Check sheet for the drawn part. Datum: minimum x, y, z corner. Units: mm. A direction names the side the tool comes from. Round coordinates to 2 decimals unless told otherwise and drop trailing zeros. Order: outer loops, then holes, each group sorted by start corner. A loop starts at its lowest first (then second) coordinate and runs counter-clockwise, first axis right, second up.
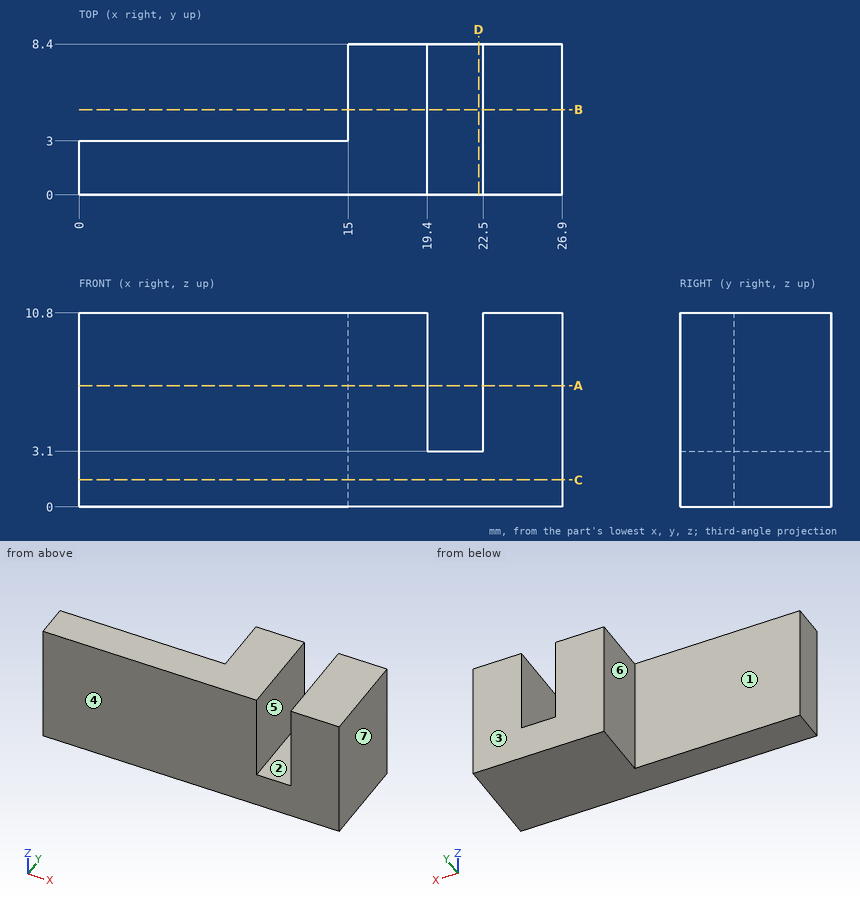
(1) Draft check along X on the marked faces 4, 5, 6 and 7. Enter one of: released by +X, released by -X, zero draft, split by the parting line, or undercut.
Returned:
face 4: zero draft
face 5: undercut
face 6: released by -X
face 7: released by +X
(2) Sectioned sample at B-B, the plane y = 4.75. Record the cut outline in (x, z), and give its area (3 significant figures).
Returned:
outline: (15, 0) - (26.9, 0) - (26.9, 10.8) - (22.5, 10.8) - (22.5, 3.1) - (19.4, 3.1) - (19.4, 10.8) - (15, 10.8) - close
area: 105 mm2
(3) Sectioned sample at A-A, the plane z = 6.75. Record the cut outline in (x, y).
Returned:
outline: (0, 0) - (19.4, 0) - (19.4, 8.4) - (15, 8.4) - (15, 3) - (0, 3) - close; (22.5, 0) - (26.9, 0) - (26.9, 8.4) - (22.5, 8.4) - close
(4) Depth check by flat-ended pin: P1, Ø3, axis at y = 4, z = 4.5, coming from the -X side; P2, Ø5.5, axis at x = 6.5, z = 7.5, coming from the +Y side. Enter the tip coordinate at first touch or a pass-through.
Returned:
P1: stops at x = 0
P2: stops at y = 3
(5) Material ranges on line 1 (X direction, y = 7, z = 9.25); line 2 (X direction, y = 1, z = 7.75); line 3 (Y direction, x = 10.25, z = 6.25), recorded low to high.
Returned:
line 1: x = 15 to 19.4, 22.5 to 26.9
line 2: x = 0 to 19.4, 22.5 to 26.9
line 3: y = 0 to 3
(6) Set-up check for the marked faces 1, 2 and 3: record each of +Z, -Z, +X, -X, +Y, -Y from which the full face is reachable in a straight line by a thin tool's end or side.
Returned:
face 1: +Z, -Z, -X, +Y
face 2: +Z, +Y, -Y
face 3: +Z, -Z, +X, -X, +Y
(7) Sectioned sample at C-C, the plane z = 1.5. Record the cut outline in (x, y).
Returned:
outline: (0, 0) - (26.9, 0) - (26.9, 8.4) - (15, 8.4) - (15, 3) - (0, 3) - close
(8) Sectioned sample at D-D, the plane x = 22.25. Record the cut outline in (y, z), and give its area (3 significant figures).
Returned:
outline: (0, 0) - (8.4, 0) - (8.4, 3.1) - (0, 3.1) - close
area: 26.0 mm2
